```python
from build123d import *
from build123d import SkipClean  # not in build123d's __all__

# Parameters (mm, degrees)
F0_R      = 4.16
F1_DEPTH  = 15
F3_DEPTH  = 100
F4_W      = 23.4
F4_H      = 8
F5_DEPTH  = 25
F7_COUNT  = 3
F9_START  = 22
F8_R      = 16.208
F8_R_2    = 13.208
F9_DEPTH  = 38
F10_R     = 12.7
F11_DEPTH = 40
F12_R     = 13.208
F13_DEPTH = 40


# Not quite as in the source:
# - a feature names something its author has since deleted; it is built from what else it names


with BuildPart() as f1:
    # F0 (on Top) → F1 (new body)
    with BuildSketch(Plane.XY):
        Polygon((-32.7, 0), (-14.7, 0), (-14.7, 50), (-14.7, 100), (-32.7, 100), (-32.7, 70), (-23.7483102828, 61), (-23.7483102828, 50), (-23.7483102828, 39), (-32.7, 30), align=None)
        with Locations((-23.7, 15)):
            Circle(F0_R, mode=Mode.SUBTRACT)
        with Locations((-23.7, 85)):
            Circle(F0_R, mode=Mode.SUBTRACT)
    extrude(amount=F1_DEPTH)

    # F2 (on face) → F3 (join)
    with BuildSketch(Plane.XZ):
        with BuildLine():
            Line((-14.7, 0), (-14.7, 15))
            ThreePointArc((-14.7, 15), (-16.5027270474, 7.5), (-14.7, 0))
        make_face()
        with BuildLine():
            ThreePointArc((-6.85, -4.3645480318), (-13.7, 7.5), (-6.85, 19.3645480318))
            Line((-6.85, 19.3645480318), (-8.2513635237, 21.7917808547))
            ThreePointArc((-8.2513635237, 21.7917808547), (-11.9675955686, 18.8629510386), (-14.7, 15))
            Line((-14.7, 15), (-14.7, 0))
            ThreePointArc((-14.7, 0), (-11.9675955686, -3.8629510386), (-8.2513635237, -6.7917808547))
            Line((-8.2513635237, -6.7917808547), (-6.85, -4.3645480318))
        make_face()
    extrude(amount=-F3_DEPTH)

    # F4 (on face) → F5 (cut)
    with BuildSketch(Plane(origin=(-32.7, 0, 0), x_dir=(0, -1, 0), z_dir=(-1, 0, 0))):
        with Locations((-84.9, 7.5)):
            Rectangle(F4_W, F4_H)
        with Locations((-15.1, 7.5)):
            Rectangle(F4_W, F4_H)
    extrude(amount=-F5_DEPTH, mode=Mode.SUBTRACT)

    # F7: F1 ×3 about axis
    f7_axis = Axis((0, 0, 7.5), (0, -1, 0))


with BuildPart() as f1_1:
    add(f1.part, clean=False)
    with SkipClean():  # cleaning this boolean's faces spoils the solid; the shape is the same uncleaned
        for i in range(1, F7_COUNT):
            add(f1.part.rotate(f7_axis, i * 360 / F7_COUNT), clean=False)

    # F8 (on Top) → F9 (join)
    with BuildSketch(Plane.XY.offset(F9_START)):
        with Locations((0, 50)):
            Circle(F8_R)
        with Locations((0, 50)):
            Circle(F8_R_2, mode=Mode.SUBTRACT)
    with SkipClean():  # cleaning this boolean's faces spoils the solid; the shape is the same uncleaned
        extrude(amount=F9_DEPTH)

    # F10 (on face) → F11 (cut)
    with BuildSketch(Plane.XY.offset(60)):
        with Locations((0, 50)):
            Circle(F10_R)
    with SkipClean():  # cleaning this boolean's faces spoils the solid; the shape is the same uncleaned
        extrude(amount=-F11_DEPTH, mode=Mode.SUBTRACT)

    # F12 (on face) → F13 (cut)
    with BuildSketch(Plane.XY.offset(60)):
        with Locations((0, 50)):
            Circle(F12_R)
    with SkipClean():  # cleaning this boolean's faces spoils the solid; the shape is the same uncleaned
        extrude(amount=-F13_DEPTH, mode=Mode.SUBTRACT)


solid = f1_1.part
```
Part model, mm, in its own coordinate system. A direction names the side the tool comes from. Round coordinates to 2 decimals unless told otherwise and drop trailing zeros. Loops run counter-clockwise (first coordinate to the right, second up) from the corner with the lowest first, then second, coordinate; pieces in that order, holes last.
Item 1: Drill centre lines: line 1 (Y direction, x = -19.5, z = 4); line 2 (Y direction, x = -23.7, z = 12.75); line 3 (Y direction, x = 0, z = 36.5). Where is each one in solid material? Low to high.
Item 2: Mould opens along Z. For faces 1 (the face through (17.3, 80.94, -10.92)), 2 (the face through (9, 50, 20)), 3 (the face through (11.97, 50.15, -13.01)) say: +Z half, -Z half, draft (parallel to the pull), parting line (faces both ways), or undercut.
Item 3: Cut at A-A, the plane y = 77. Give the cut face in (x, z), then the cut area to 4 significant figures.
Item 4: 3-axis set-ups, long thin cutter, end or side, ignore diameter. For faces 4 (the face through (-22, 51, 0)), 5 (the face through (-23, 26.8, 7)), 6 (the face through (12.806, 15.264, 21.681)): which of +Z, -Z, +X, -X, +Y, -Y reach the whole face in a straight line?
Item 5: Cut at C-C, the plane z = 41.5. Give the cut face in (x, y).
Item 6: Drop flat-ended pins along their axis: P1, Ø7.5, axis at y = 50.5, z = 4, coming from the -X side; P2, Ø10, axis at y = 47, z = 40.5, coming from the -X side; P3, Ø3, axis at x = 10, y = 70, coming from the +Z side. Give the stop position or say it passes through.
Item 7: Cut at D-D, the plane y = 50. Give the cut face in (x, z).
Item 8: Cut at B-B, the plane z = 13. Give the cut face in (x, y), then the cut area to 3 significant figures.
A:
1. line 1: y = 0 to 3.4, 26.8 to 73.2, 96.6 to 100
1. line 2: y = 0 to 10.84, 19.16 to 80.84, 89.16 to 100
1. line 3: y = 33.79 to 36.79, 63.21 to 66.21
2. face 1: undercut
2. face 2: +Z half
2. face 3: -Z half
3. outline: (-32.7, 0) - (-14.7, 0) arc R16.5 ccw to (0.85, -8.98) - (9.85, -24.57) - (12.89, -22.82) - (3.09, -5.85) arc R13.7 cw to (-13.1, 3.5) - (-32.7, 3.5) - close; (-32.7, 11.5) - (-13.1, 11.5) arc R13.7 cw to (3.09, 20.85) - (12.89, 37.82) - (9.85, 39.57) - (0.85, 23.98) arc R16.5 ccw to (-14.7, 15) - (-32.7, 15) - close; (10.02, -1.85) - (19.81, -18.82) - (22.85, -17.07) - (13.85, -1.48) arc R16.5 ccw to (13.85, 16.48) - (22.85, 32.07) - (19.81, 33.82) - (10.02, 16.85) arc R13.7 cw to start
3. area: 560.5 mm2
4. face 4: -Z, -X, +Y, -Y
4. face 5: -X
4. face 6: none
5. outline: circle Ø32.42 at (0, 50); hole circle Ø26.42 at (0, 50)
6. P1: stops at x = -23.75
6. P2: stops at x = -16.21
6. P3: stops at z = 39.57
7. outline: (-23.75, 0) - (-14.7, 0) arc R16.5 ccw to (0.85, -8.98) - (5.38, -16.82) - (18.37, -9.32) - (13.85, -1.48) arc R16.5 ccw to (13.85, 16.48) - (18.37, 24.32) - (16.21, 25.56) - (16.21, 60) - (13.21, 60) - (13.21, 20) - (5.61, 20) arc R13.7 cw (long way) to (-5.61, 20) - (-10.77, 20) arc R16.5 ccw to (-14.7, 15) - (-23.75, 15) - close; (-16.21, 22) - (-13.21, 22) - (-13.21, 60) - (-16.21, 60) - close
8. outline: (-32.7, 0) - (-12.55, 0) - (-12.55, 100) - (-32.7, 100) - (-32.7, 70) - (-23.75, 61) - (-23.75, 39) - (-32.7, 30) - close; (12.55, 0) - (15.56, 0) - (15.56, 100) - (12.55, 100) - close; hole circle Ø8.32 at (-23.7, 15); hole circle Ø8.32 at (-23.7, 85)
8. area: 1,930 mm2
